For this review, take the finished solid that the model builds, in its own axes (mm). A direction names the side the tool comes from. Coordinates: 2 decimals unless noted, no trailing zeros. Loops run counter-clockwise (first coordinate to the right, second up) from the corner with the lowest first, then second, coordinate; pieces in that order, holes last. Notation, with made-up numbers: (26, 74) - (72, 74) arc R24 cw to (72, 90) - close; hole circle Ø4 at (21.25, 4). An arc over 180 degrees is marked (long way). Answer as a JSON object with one key per item and string values. Group by question number.
Item 1: We need section A-A (y = 50). Give the boundary of the cut face in (x, z), then the cut area to 3 significant figures.
Item 2: We need section C-C (y = 56.5). Give the boundary of the cut face in (x, z).
Item 3: We need section B-B (x = 0). Give the boundary of the cut face in (y, z), then the cut area to 4 significant figures.
Item 4: We need section D-D (z = 0). Give the boundary of the cut face in (x, y).
Item 5: Tool access review of faces 5 (the cylindrical face through (0, 2, 2)), 6 (the flat face through (0, 5, 0)), 7 (the cylindrical face through (12.65, 28.94, -12.68)): name each direction out of +Z, -Z, +X, -X, +Y, -Y from which nothing blocks a thin tool from reaching the whole face with its end or side.
Item 6: Mouldability with a two-part tool opening along X and no side actions: class faces 1 (the cylindrical face through (0, 53, -12)), 2 (the flat face through (-0.1, 0, 2.4)), 3 (the cylindrical face through (-12.65, 28.94, 9.68)), 4 (the flat face through (13.25, 29, -2)) as released by +X, released by -X, zero draft, split by the parting line, or undercut.
Item 7: Clearance check with flat-ended pins moving along their axes: pin 1 (3 mm diameter, centred on x = 0, z = 0, fed in from +Y); pin 2 (3.5 mm diameter, centred on x = 0, y = 17, fed in from +Z); pin 3 (3 mm diameter, centred on x = -7.5, z = -4.5, fed in from +Y). State where each tip first meets the part, or that it passes through.
Item 8: To check wall thickness, follow line 1 (Y direction, x = 0, z = -12.15); line 2 (X direction, y = 43.5, z = -8); line 3 (Y direction, x = -1.5, z = 6). State the ranges of each line that lie inside material, in increasing order.
from build123d import *

# Parameters (mm, degrees)
BOSS_EXTRUDE1_DEPTH = 60
SKETCH2_W           = 20.5
SKETCH2_H           = 20.5
BOSS_EXTRUDE2_DEPTH = 3
SKETCH3_R           = 2
BOSS_EXTRUDE3_DEPTH = 5
SKETCH4_R           = 3
CUT_EXTRUDE1_DEPTH  = 23.5


with BuildPart() as part:
    # Sketch1 → Boss-Extrude1 (new body)
    with BuildSketch(Plane(origin=(0, 0, 0), x_dir=(1, 0, 0), z_dir=(0, 1, 0))):
        with BuildLine():
            Line((-13.25, 11.25), (-13.25, -8.25))
            ThreePointArc((-13.25, -8.25), (-12.664213562, -9.664213562), (-11.25, -10.25))
            Line((-11.25, -10.25), (-10.25, -10.25))
            Line((-10.25, -10.25), (-10.25, 10.25))
            Line((-10.25, 10.25), (10.25, 10.25))
            Line((10.25, 10.25), (10.25, -10.25))
            Line((10.25, -10.25), (11.25, -10.25))
            ThreePointArc((11.25, -10.25), (12.664213562, -9.664213562), (13.25, -8.25))
            Line((13.25, -8.25), (13.25, 11.25))
            ThreePointArc((13.25, 11.25), (12.664213562, 12.664213562), (11.25, 13.25))
            Line((11.25, 13.25), (-11.25, 13.25))
            ThreePointArc((-11.25, 13.25), (-12.664213562, 12.664213562), (-13.25, 11.25))
        make_face()
    extrude(amount=BOSS_EXTRUDE1_DEPTH)

    # Sketch2 → Boss-Extrude2 (add)
    with BuildSketch(Plane.XZ):
        with BuildLine():
            ThreePointArc((-11.25, 10.25), (-12.664213562, 9.664213562), (-13.25, 8.25))
            Line((-13.25, 8.25), (-13.25, -11.25))
            ThreePointArc((-13.25, -11.25), (-12.664213562, -12.664213562), (-11.25, -13.25))
            Line((-11.25, -13.25), (11.25, -13.25))
            ThreePointArc((11.25, -13.25), (12.664213562, -12.664213562), (13.25, -11.25))
            Line((13.25, -11.25), (13.25, 8.25))
            ThreePointArc((13.25, 8.25), (12.664213562, 9.664213562), (11.25, 10.25))
            Line((11.25, 10.25), (10.25, 10.25))
            Line((10.25, 10.25), (10.25, -10.25))
            Line((10.25, -10.25), (-10.25, -10.25))
            Line((-10.25, -10.25), (-10.25, 10.25))
            Line((-10.25, 10.25), (-11.25, 10.25))
        make_face()
        Rectangle(SKETCH2_W, SKETCH2_H)
    extrude(amount=BOSS_EXTRUDE2_DEPTH)

    # Sketch3 → Boss-Extrude3 (add)
    with BuildSketch(Plane(origin=(0, 0, 0), x_dir=(1, 0, 0), z_dir=(0, 1, 0))):
        Circle(SKETCH3_R)
    extrude(amount=BOSS_EXTRUDE3_DEPTH)

    # Sketch4 → Cut-Extrude1 (cut)
    with BuildSketch(Plane(origin=(0, 0, -13.25), x_dir=(-1, 0, 0), z_dir=(0, 0, -1))):
        with Locations((0, 50)):
            Circle(SKETCH4_R)
        with Locations((0, 17)):
            Circle(SKETCH4_R)
    extrude(amount=-CUT_EXTRUDE1_DEPTH, mode=Mode.SUBTRACT)


solid = part.part
Check sheet entries:
{
 "1": {"outline": "(-13.25, -11.25) arc R2 ccw to (-11.25, -13.25) - (-3, -13.25) - (-3, -10.25) - (-10.25, -10.25) - (-10.25, 10.25) - (-11.25, 10.25) arc R2 ccw to (-13.25, 8.25) - close; (3, -13.25) - (11.25, -13.25) arc R2 ccw to (13.25, -11.25) - (13.25, 8.25) arc R2 ccw to (11.25, 10.25) - (10.25, 10.25) - (10.25, -10.25) - (3, -10.25) - close", "area": "181 mm2"},
 "2": {"outline": "(-13.25, -11.25) arc R2 ccw to (-11.25, -13.25) - (11.25, -13.25) arc R2 ccw to (13.25, -11.25) - (13.25, 8.25) arc R2 ccw to (11.25, 10.25) - (10.25, 10.25) - (10.25, -10.25) - (-10.25, -10.25) - (-10.25, 10.25) - (-11.25, 10.25) arc R2 ccw to (-13.25, 8.25) - close"},
 "3": {"outline": "(-3, -13.25) - (14, -13.25) - (14, -10.25) - (0, -10.25) - (0, -2) - (5, -2) - (5, 2) - (0, 2) - (0, 10.25) - (-3, 10.25) - close; (20, -13.25) - (47, -13.25) - (47, -10.25) - (20, -10.25) - close; (53, -13.25) - (60, -13.25) - (60, -10.25) - (53, -10.25) - close", "area": "234.5 mm2"},
 "4": {"outline": "(-13.25, -3) - (13.25, -3) - (13.25, 60) - (10.25, 60) - (10.25, 0) - (2, 0) - (2, 5) - (-2, 5) - (-2, 0) - (-10.25, 0) - (-10.25, 60) - (-13.25, 60) - close"},
 "5": {"face 5": "+Y", "face 6": "+Z, +Y", "face 7": "-Z, +X, +Y, -Y"},
 "6": {"face 1": "undercut", "face 2": "undercut", "face 3": "released by -X", "face 4": "released by +X"},
 "7": {"pin 1": "stops at y = 5", "pin 2": "passes through", "pin 3": "stops at y = 0"},
 "8": {"line 1": "y = -3 to 14, 20 to 47, 53 to 60", "line 2": "x = -13.25 to -10.25, 10.25 to 13.25", "line 3": "y = -3 to 0"}
}
